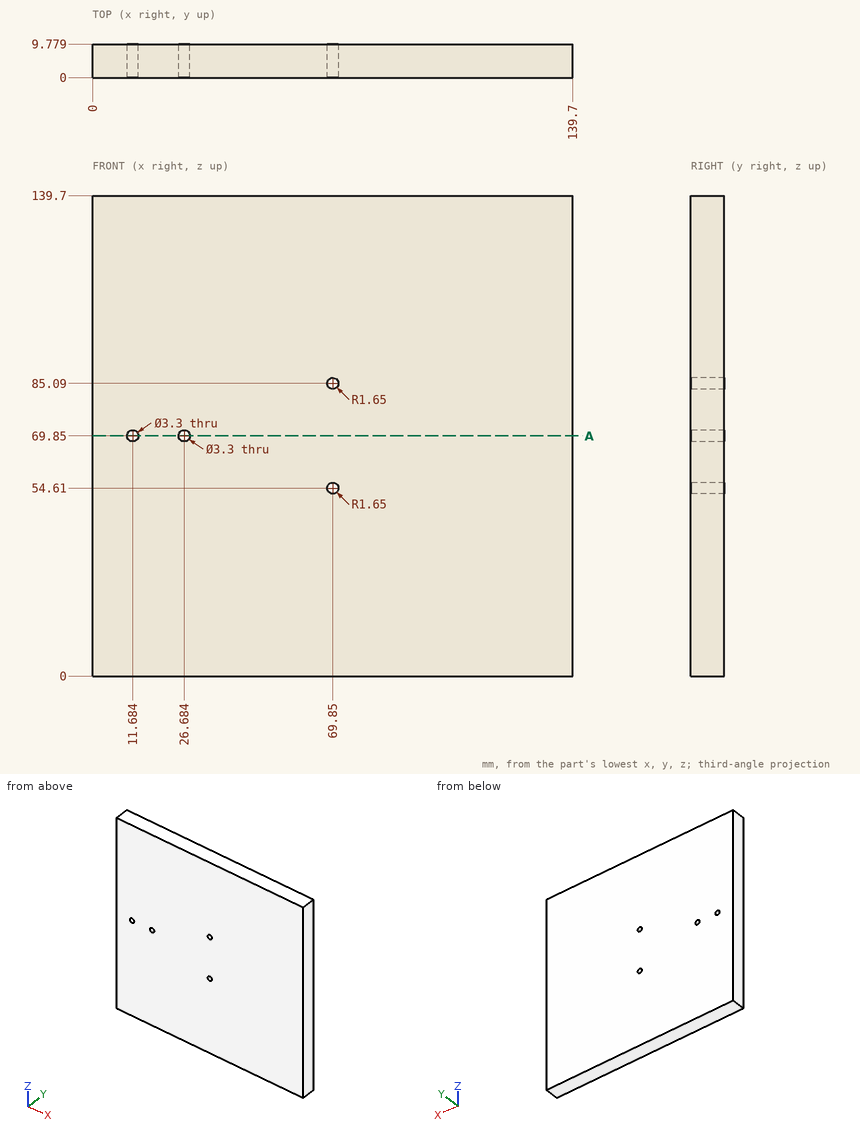
Design review of the part shown in the three views and the two pictorial views. Dimensions are in mm from the part's minimum x, y and z. Round coordinates to 2 decimals unless told otherwise and drop trailing zeros. Loops run counter-clockwise (first coordinate to the right, second up) from the corner with the lowest first, then second, coordinate; pieces in that order, holes last. Notation, with made-up numbers: (0, 51.5) - (33, 51.5) arc R24 cw to (33, 62.5) - close; hole circle Ø8 at (-13.5, -20.75). An arc over 180 degrees is marked (long way). Write each question's results on one line, items separated by ' | '. Start each with the question number.
Q1. Insertion check: P1, Ø2, axis at x = 11.684, z = 69.85, coming from the -Y side; P2, Ø4, axis at x = 47, y = 2, coming from the -Z side. Each pin has a flat end and moves straight along its axis. Give the tip position at first contact, or say it passes through.
Q2. Wall thickness on line 1 along X through (y, z) = (4.75, 69.85); line 2 along Z through (x, y) = (28, 1.5); line 3 along Z through (x, y) = (25.5, 0.5): over which ranges is each line inside the solid? List them lowest first. Write a range as [from, to].
Q3. Take a section at A-A on z = 69.85. Give the boundary of the cut face in (x, y), plus the area to 3 significant figures.
Data:
1) P1: passes through | P2: stops at z = 0
2) line 1: x = [0, 10.03], [13.33, 25.03], [28.33, 139.7] | line 2: z = [0, 68.85], [70.85, 139.7] | line 3: z = [0, 68.7], [71, 139.7]
3) outline: (0, 0) - (10.03, 0) - (10.03, 9.78) - (0, 9.78) - close; (13.33, 0) - (25.03, 0) - (25.03, 9.78) - (13.33, 9.78) - close; (28.33, 0) - (139.7, 0) - (139.7, 9.78) - (28.33, 9.78) - close | area: 1,300 mm²
